from build123d import *

# Parameters (mm, degrees)
F0_W     = 195
F0_H     = 145
F0_W_2   = 180
F0_H_2   = 130
F0_W_3   = 175
F0_H_3   = 125
F1_DEPTH = 5
F2_DEPTH = 1
F3_DEPTH = 0.2


with BuildPart() as f1:
    # F0 (on Top) → F1 (new body)
    with BuildSketch(Plane.XY):
        Rectangle(F0_W, F0_H)
        Rectangle(F0_W_2, F0_H_2, mode=Mode.SUBTRACT)
        Rectangle(F0_W_2, F0_H_2)
        Rectangle(F0_W_3, F0_H_3, mode=Mode.SUBTRACT)
    extrude(amount=F1_DEPTH)

    # F0 (on Top) → F2 (join)
    with BuildSketch(Plane.XY):
        Rectangle(F0_W, F0_H)
        Rectangle(F0_W_2, F0_H_2, mode=Mode.SUBTRACT)
        Rectangle(F0_W_2, F0_H_2)
        Rectangle(F0_W_3, F0_H_3, mode=Mode.SUBTRACT)
    extrude(amount=-F2_DEPTH)

    # F0 (on Top) → F3 (cut)
    with BuildSketch(Plane.XY):
        Rectangle(F0_W_2, F0_H_2)
        Rectangle(F0_W_3, F0_H_3, mode=Mode.SUBTRACT)
    extrude(amount=F3_DEPTH, mode=Mode.SUBTRACT)


solid = f1.part
Geometry check sheet. Reference: the model listing, model coordinates, mm. A direction names the side the tool comes from. Round coordinates to 2 decimals unless told otherwise and drop trailing zeros. Order: outer loops, then holes, each group sorted by start corner. A loop starts at its lowest first (then second) coordinate and runs counter-clockwise, first axis right, second up. Notation, with made-up numbers: M 25.5,47 L 49.5,47 A21 cw 49.5,57 Z; hole C 5,-21 d8. An arc over 180 degrees is marked long. Answer in a Markdown table with one row per item.
(1) Sectioned sample at C-C, the plane z = 4. Record the cut outline in (x, y), and give its area (3 significant figures).
Responses:
| item | result |
|---|---|
| outline | M -97.5,-72.5 L 97.5,-72.5 L 97.5,72.5 L -97.5,72.5 Z; hole M -87.5,-62.5 L 87.5,-62.5 L 87.5,62.5 L -87.5,62.5 Z |
| area | 6,400 mm² |
(2) Scan lines: probe 1 along Y at (x, z) = (56, 4.65); probe 2 along X at (y, z) = (-51, -0.45). Record each from-to range of solid material in increasing order. Write a range as from..to.
Responses:
| item | result |
|---|---|
| probe 1 | y = -72.5..-62.5, 62.5..72.5 |
| probe 2 | x = -97.5..-87.5, 87.5..97.5 |
(3) Sectioned sample at A-A, the plane y = -38. Record the cut outline in (x, z), and give its area (3 significant figures).
Responses:
| item | result |
|---|---|
| outline | M -97.5,-1 L -87.5,-1 L -87.5,0 L -90,0 L -90,0.2 L -87.5,0.2 L -87.5,5 L -97.5,5 Z; M 87.5,-1 L 97.5,-1 L 97.5,5 L 87.5,5 L 87.5,0.2 L 90,0.2 L 90,0 L 87.5,0 Z |
| area | 119 mm² |
(4) Tool access check on faces 1 (the face through (87.5, -1, 3)), 2 (the face through (0, 63, 0.2)), 3 (the face through (97.5, -1, 2)). Record the directions out of +Z, -Z, +X, -X, +Y, -Y that give a thin tool (end or side, any length) a straight path to the whole face; none if there is none.
Responses:
| item | result |
|---|---|
| face 1 | +Z, -Z |
| face 2 | none |
| face 3 | +Z, -Z, +X, +Y, -Y |
(5) Sectioned sample at B-B, the plane x = 14. Record the cut outline in (y, z), and give its area (3 significant figures).
Responses:
| item | result |
|---|---|
| outline | M -72.5,-1 L -62.5,-1 L -62.5,0 L -65,0 L -65,0.2 L -62.5,0.2 L -62.5,5 L -72.5,5 Z; M 62.5,-1 L 72.5,-1 L 72.5,5 L 62.5,5 L 62.5,0.2 L 65,0.2 L 65,0 L 62.5,0 Z |
| area | 119 mm² |
(6) Draft check along Y on faces 4 (the face through (-1, -72.5, 2)), 5 (the face through (-1, 72.5, 2)), 6 (the face through (-97.5, -1, 2)), 7 (the face through (0, 63, 0)). Enter one of: released by +Y, released by -Y, zero draft, split by the parting line, or undercut.
Responses:
| item | result |
|---|---|
| face 4 | released by -Y |
| face 5 | released by +Y |
| face 6 | zero draft |
| face 7 | undercut |
